Can you work these out from the drawing? Everything is in mm from the part's minimum corner. Give positions to 0.01 mm unless a question says otherwise; leave off trailing zeros. Write each loop counter-clockwise with the first axis right and the second up, starting at its lowest first coordinate (ties: lowest second). Pieces come first, ordered by that corner, then holes. Notation, with made-up numbers: (64.25, 66.5) - (83.25, 66.5) arc R7 ccw to (83.25, 74.5) - close; hole circle Ø8 at (82.5, 1). An arc over 180 degrees is marked (long way). Write each question's results on one line, items separated by ' | '. Start each with the question number.
Item 1: Suppose I cut it at D-D on z = 1.05. List the corners of the cut face in (x, y) for me.
Item 2: Will these pins go through, and if not, where does the flat tip stop? P1, Ø1.2, axis at y = 48.5, z = 1, coming from the -X side; P2, Ø1, axis at x = 41.5, z = 2, coming from the -Y side; P3, Ø1.2, axis at x = 47.5, z = 1, coming from the -Y side; P4, Ø2, axis at x = 11.1, y = 24.9, coming from the -Z side.
Item 3: Please list where these lines run through material, in increasing order: line 1 along X through (y, z) = (24.5, 0.9); line 2 along Y through (x, z) = (24.9, 0.75); line 3 along X through (y, z) = (17.5, 0.8) (1 decimal).
Item 4: Suppose I cut it at B-B on x = 18. List the corners of the cut face in (y, z) for me.
Item 5: Suppose I cut it at C-C on y = 30. List the corners of the cut face in (x, z) for me.
Item 6: Suppose I cut it at A-A on y = 24.9. List the corners of the cut face in (x, z) for me, then the cut area to 3 significant figures.
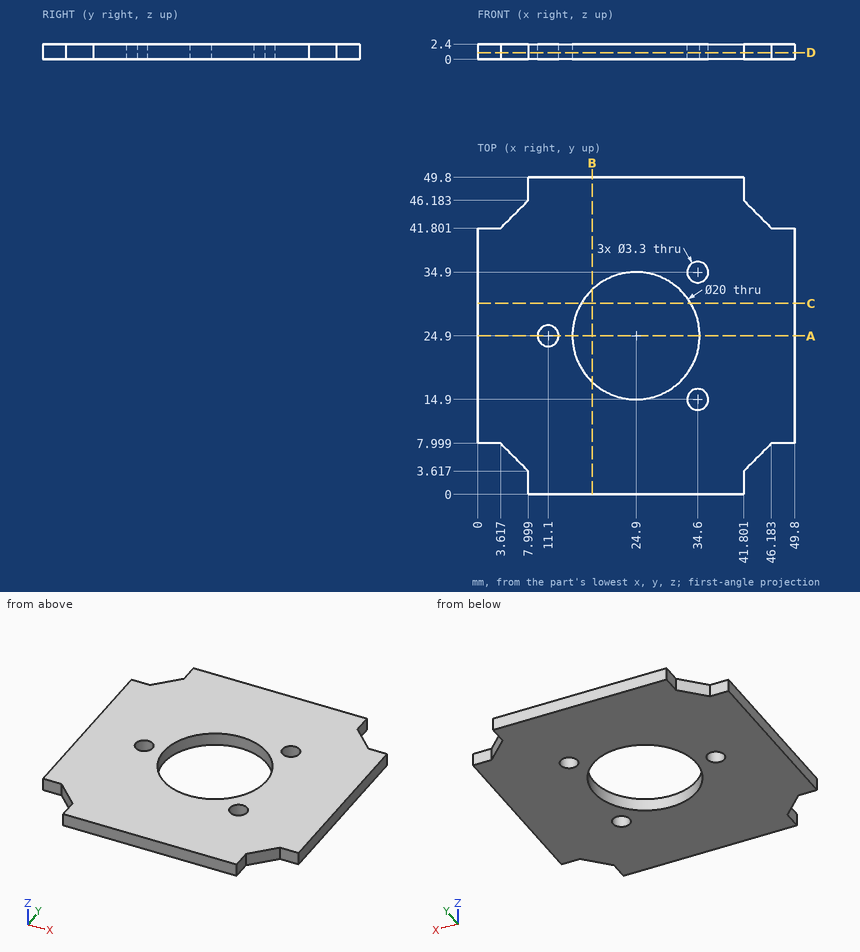
Checked values:
1) outline: (0, 8) - (3.62, 8) - (8, 3.62) - (8, 0) - (41.8, 0) - (41.8, 3.62) - (46.18, 8) - (49.8, 8) - (49.8, 41.8) - (46.18, 41.8) - (41.8, 46.18) - (41.8, 49.8) - (8, 49.8) - (8, 46.18) - (3.62, 41.8) - (0, 41.8) - close; hole circle Ø3.3 at (11.1, 24.9); hole circle Ø20 at (24.9, 24.9); hole circle Ø3.3 at (34.6, 14.9); hole circle Ø3.3 at (34.6, 34.9)
2) P1: stops at x = 8 | P2: stops at y = 0 | P3: stops at y = 8 | P4: passes through
3) line 1: x = 0 to 9.5, 12.7 to 14.91, 34.89 to 49.8 | line 2: y = 0 to 14.9, 34.9 to 49.8 | line 3: x = 0 to 18.2, 31.6 to 49.8
4) outline: (0, 0) - (17.66, 0) - (17.66, 2.4) - (0, 2.4) - close; (32.14, 0) - (49.8, 0) - (49.8, 2.4) - (32.14, 2.4) - close
5) outline: (0, 0) - (16.3, 0) - (16.3, 2.4) - (0, 2.4) - close; (33.5, 0) - (49.8, 0) - (49.8, 2.4) - (33.5, 2.4) - close
6) outline: (0, 0) - (9.45, 0) - (9.45, 2.4) - (0, 2.4) - close; (12.75, 0) - (14.9, 0) - (14.9, 2.4) - (12.75, 2.4) - close; (34.9, 0) - (49.8, 0) - (49.8, 2.4) - (34.9, 2.4) - close | area: 63.6 mm^2
